```python
from build123d import *

# Parameters (mm, degrees)
SKETCH_W         = 4.6
SKETCH_H         = 4.6
PAD_DEPTH        = 1.04
SKETCH001_W      = 0.47
SKETCH001_H      = 3.5
PAD001_DEPTH     = 0.42
CHAMFER_SIZE     = 0.6
SKETCH002_R      = 0.9
PAD002_DEPTH     = 0.45
REVOLUTION_ANGLE = 180
SKETCH004_W      = 4.6
SKETCH004_H      = 4.6
PAD003_DEPTH     = 0.6
CHAMFER001_SIZE  = 0.5
SKETCH005_W      = 3.6
SKETCH005_H      = 1.412588
PAD004_DEPTH     = 0.96
CHAMFER002_SIZE  = 0.4
CHAMFER003_SIZE  = 0.4


with BuildPart() as part:
    # Sketch → Pad (new body)
    with BuildSketch(Plane.XZ):
        with Locations((0, 2.3)):
            Rectangle(SKETCH_W, SKETCH_H)
    extrude(amount=PAD_DEPTH)

    # Sketch001 → Pad001 (new body)
    with BuildSketch(Plane.XZ.offset(1.04)):
        with Locations((0, -1.75)):
            Rectangle(SKETCH001_W, SKETCH001_H)
        Polygon((1.635, 0), (1.635, -0.42), (2.235, -0.42), (2.235, -3.5), (1.765, -3.5), (1.765, -1), (1.165, -1), (1.165, 0), align=None)
        Polygon((-1.635, 0), (-1.635, -0.42), (-2.235, -0.42), (-2.235, -3.5), (-1.765, -3.5), (-1.765, -1), (-1.165, -1), (-1.165, 0), align=None)
    extrude(amount=-PAD001_DEPTH)

    # Chamfer
    chamfer_edges = [part.edges().sort_by_distance(p)[0] for p in [
        (0, 0, 4.6),
        (2.3, 0, 2.3),
        (-2.3, 0, 2.3),
        (0, 0, 0),
    ]]
    chamfer(chamfer_edges, length=CHAMFER_SIZE)

    # Sketch002 → Pad002 (new body)
    with BuildSketch(Plane.XZ.offset(1.04)):
        with Locations((0, 2.8)):
            Circle(SKETCH002_R)
    extrude(amount=PAD002_DEPTH)

    # Sketch003 → Revolution (revolve)
    with BuildSketch(Plane.XZ.offset(1.49)):
        with BuildLine():
            ThreePointArc((-1.1e-05, 3.7), (-0.9, 2.8), (-1.1e-05, 1.9))
            Line((-1.1e-05, 3.7), (-1.1e-05, 1.9))
        make_face()
    revolve(axis=Axis((0, -1.49, 0), (0, 0, 1)), revolution_arc=REVOLUTION_ANGLE)

    # Sketch004 → Pad003 (new body)
    with BuildSketch(Plane.XZ.offset(1.04)):
        with Locations((0, 2.3)):
            Rectangle(SKETCH004_W, SKETCH004_H)
    extrude(amount=PAD003_DEPTH)

    # Chamfer001
    chamfer001_edges = [part.edges().sort_by_distance(p)[0] for p in [
        (0, -1.64, 4.6),
        (2.3, -1.64, 2.3),
        (0, -1.64, 0),
        (-2.3, -1.64, 2.3),
    ]]
    chamfer(chamfer001_edges, length=CHAMFER001_SIZE)

    # Sketch005 → Pad004 (new body)
    with BuildSketch(Plane.XZ.offset(1.64)):
        with Locations((0, 1.206294)):
            Rectangle(SKETCH005_W, SKETCH005_H)
    extrude(amount=PAD004_DEPTH)

    # Chamfer002
    chamfer002_edges = [part.edges().sort_by_distance(p)[0] for p in [
        (0, -2.6, 1.912588),
        (0, -2.6, 0.5),
        (-1.8, -2.6, 1.206294),
        (1.8, -2.6, 1.206294),
    ]]
    chamfer(chamfer002_edges, length=CHAMFER002_SIZE)

    # Chamfer003
    chamfer003_edges = [part.edges().sort_by_distance(p)[0] for p in [
        (0, -2.2, 1.912588),
        (1.8, -2.2, 1.206294),
        (0, -2.2, 0.5),
        (-1.8, -2.2, 1.206294),
    ]]
    chamfer(chamfer003_edges, length=CHAMFER003_SIZE)


solid = part.part
```
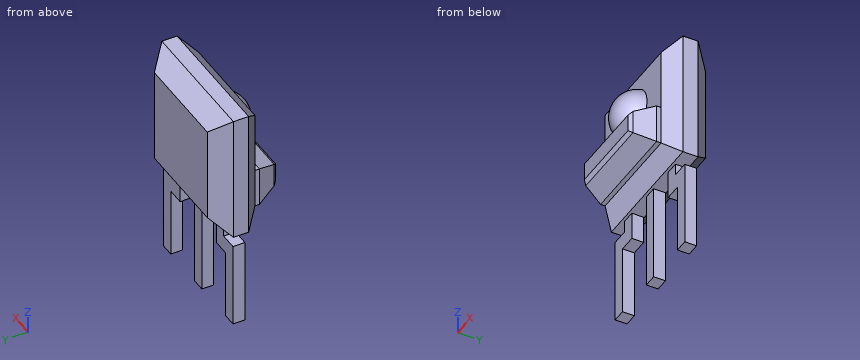
Here's how the part is built. I have some questions about the finished solid (model axes, mm). Round coordinates to 2 decimals unless told otherwise and drop trailing zeros. Loops run counter-clockwise (first coordinate to the right, second up) from the corner with the lowest first, then second, coordinate; pieces in that order, holes last. Notation, with made-up numbers: (-23, 25.5) -> (10, 25.5) arc R35 cw to (10, 64.5) -> close; hole circle Ø4 at (21, 23). An arc over 180 degrees is marked (long way). Answer as CSV lines item,"result". Start each with the question number.
1. I'm going to push flat-ended pins straight in: P1, Ø0.9, axis at x = -1.5, z = -1, coming from the +Y side; P2, Ø1.2, axis at x = -1.5, z = -1.5, coming from the -Y side; P3, Ø1, axis at x = 2, y = -2, coming from the +Z side. Where does each tip first touch, or does it pass through?
2. I need wall thicknesses on probe 1 along Y at (x, z) = (0.2, -0.5); probe 2 along Y at (x, z) = (1.6, 3); probe 3 along Z at (x, y) = (0.65, -1.9). Which ranges of each line are inside material? Lowest first, please. Write a range as from..to.
3. Imagine slicing it at D-D on y = -0.85. Write out the boundary of the cut face in (x, z) (3 decimals).
4. Imagine slicing it at B-B on z = 4.25. Write out the boundary of the cut face in (x, y).
5. Imagine slicing it at A-A on z = -2. Write out the boundary of the cut face in (x, y) (3 decimals).
6. Imagine slicing it at C-C on y = -2.3. Write out the boundary of the cut face in (x, z), plus the area to 3 significant figures.
Solution:
1,P1,"y = -0.62"
1,P2,"y = -1.04"
1,P3,"z = 4.24"
2,probe 1,"-1.04..-0.62"
2,probe 2,"-1.64..0"
2,probe 3,"0.54..1.87, 2.33..3.27"
3,outline,"(-2.3, 0) -> (-1.635, 0) -> (-1.635, -0.42) -> (-2.235, -0.42) -> (-2.235, -3.5) -> (-1.765, -3.5) -> (-1.765, -1) -> (-1.165, -1) -> (-1.165, 0) -> (-0.235, 0) -> (-0.235, -3.5) -> (0.235, -3.5) -> (0.235, 0) -> (1.165, 0) -> (1.165, -1) -> (1.765, -1) -> (1.765, -3.5) -> (2.235, -3.5) -> (2.235, -0.42) -> (1.635, -0.42) -> (1.635, 0) -> (2.3, 0) -> (2.3, 4.6) -> (-2.3, 4.6) -> close"
4,outline,"(-2.3, -1.14) -> (-1.95, -1.49) -> (1.95, -1.49) -> (2.3, -1.14) -> (2.3, -0.6) -> (1.95, -0.25) -> (-1.95, -0.25) -> (-2.3, -0.6) -> close"
5,outline,"(-2.235, -1.04) -> (-1.765, -1.04) -> (-1.765, -0.62) -> (-2.235, -0.62) -> close; (-0.235, -1.04) -> (0.235, -1.04) -> (0.235, -0.62) -> (-0.235, -0.62) -> close; (1.765, -1.04) -> (2.235, -1.04) -> (2.235, -0.62) -> (1.765, -0.62) -> close"
6,outline,"(-1.59, 0.71) -> (1.59, 0.71) -> (1.59, 1.71) -> (-1.59, 1.71) -> close; circle Ø0.78 at (0, 2.8)"
6,area,"3.66 mm²"
